For this review, take the finished solid that the model builds, in its own axes (mm). Face numbers are marked on the shaded views. Coordinates: 2 decimals unless noted, no trailing zeros. Order: outer loops, then holes, each group sorted by start corner. A loop starts at its lowest first (then second) coordinate and runs counter-clockwise, first axis right, second up.
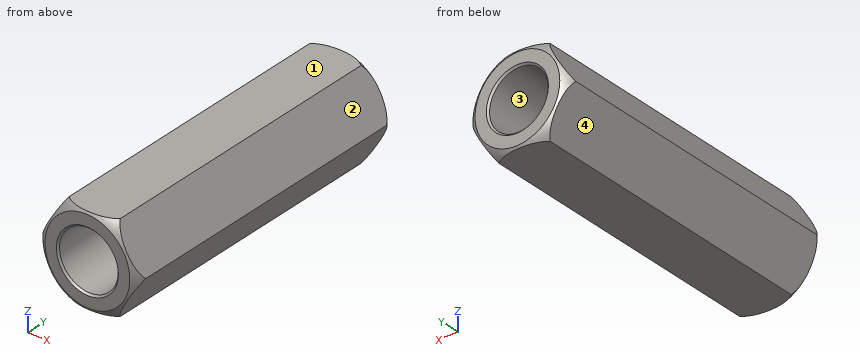
Autodesk Inventor part; units mm, degrees
ref_plane "YZ Plane" through (0, 0, 0) normal (1, 0, 0) x (0, 1, 0)
ref_plane "XZ Plane" through (0, 0, 0) normal (0, 1, 0) x (-1, 0, 0)
ref_plane "XY Plane" through (0, 0, 0) normal (0, 0, 1) x (1, 0, 0)
sketch "Sketch1" plane through (0, 0, 0) normal (0, 1, 0) x (-1, 0, 0)
  line L0 (-1.8331, -3.175) -> (-3.6662, 0)
  line L1 (-3.6662, 0) -> (-1.8331, 3.175)
  line L2 (-1.8331, 3.175) -> (1.8331, 3.175)
  line L3 (1.8331, 3.175) -> (3.6662, 0)
  line L4 (3.6662, 0) -> (1.8331, -3.175)
  line L5 (1.8331, -3.175) -> (-1.8331, -3.175)
  point P0 (0, 0)
  point P1 (0, 0)
  dimension "d0" = 6.35
extrude "Body" add sketch "Sketch1" along normal blind 22.225
sketch "Sketch2" plane through (0, 22.225, 0) normal (0, 1, 0) x (1, 0, 0)
  circle A0 centre (0, 0) radius 2.0955
  dimension "d3" = 4.191
extrude "Hole 2" cut sketch "Sketch2" against normal blind 12.7
sketch "Sketch3" plane through (0, 0, 0) normal (0, -1, 0) x (1, 0, 0)
  circle A0 centre (0, 0) radius 2.0955
  dimension "d6" = 4.191
extrude "Hole 1" cut sketch "Sketch3" against normal blind 12.7
chamfer "Hole 2 Chamfer 1" distance 0.127 distance2 0.1244 1 edges at (-2.0955, 22.225, 0) measured on face at (0.0842, 22.225, 2.8101)
chamfer "Hole 1 Chamfer 1" distance 0.127 distance2 0.1244 1 edges at (-2.0955, 0, 0) measured on face at (-0.0842, 0, 2.8101)
sketch "Sketch4" plane through (0, 0, 0) normal (0, 0, 1) x (1, 0, 0)
  line L0 (1.8331, 22.225) -> (-1.8331, 22.225)
  line L1 (0, 22.225) -> (-3.0353, 22.225)
  line L2 (-3.6662, 22.225) -> (-1.8331, 22.225)
  line L3 (-3.6662, 0) -> (-3.6662, 22.225)
  arc A0 (-3.0353, 22.225) -> (-3.6662, 21.59) centre (-2.2234, 20.7874) ccw
  line L4 (-3.6662, 21.59) -> (-6.3588, 24.1897)
  line L5 (-6.3588, 24.1897) -> (0, 22.225)
  line L6 (0, 22.225) -> (0, 75.889)
  point P0 (0, 0)
  dimension "d15" = 3.0353
  dimension "d16" = 1.651
  dimension "d17" = 0.635
revolve "Hole 2 Chamfer 2" cut sketch "Sketch4" angle 360 about axis through (0, 22.225, 0) along (0, 1, 0)
sketch "Sketch5" plane through (0, 0, 0) normal (0, 0, 1) x (1, 0, 0)
  line L0 (0, 0) -> (-3.0353, 0)
  line L1 (1.8331, 0) -> (-1.8331, 0)
  line L2 (-3.6662, 0) -> (-3.6662, 22.225)
  arc A0 (-3.6662, 0.635) -> (-3.0353, 0) centre (-2.2234, 1.4376) ccw
  line L3 (0, 0) -> (0, -2.1986)
  line L4 (-3.6662, 0.635) -> (-4.1154, -0.8715)
  line L5 (-4.1154, -0.8715) -> (0, 0)
  point P0 (-3.6662, 21.59)
  dimension "d19" = 3.0353
  dimension "d20" = 1.651
  dimension "d21" = 0.635
revolve "Hole 1 Chamfer 2" cut sketch "Sketch5" angle 360 about axis through (0, 0, 0) along (0, -1, 0)
chamfer "Hole 2 Chamfer 1 For Short" [suppressed]
sketch "Sketch7" plane through (0, 0, 0) normal (0, 0, 1) x (1, 0, 0)
  line L0 (0, 22.2254) -> (3.0353, 22.225)
  line L1 (3.6662, 22.225) -> (1.8331, 22.225)
  line L2 (3.6662, 0.635) -> (3.6662, 22.225)
  arc A0 (3.6662, 21.59) -> (3.0353, 22.225) centre (2.2234, 20.7874) ccw
  line L3 (3.6662, 21.59) -> (4.2663, 23.1282)
  line L4 (4.2663, 23.1282) -> (0, 22.2254)
  line L5 (0, 24.0311) -> (0, 22.2254)
  line L6 (1.8331, 22.225) -> (-1.8331, 22.225)
  point P0 (0, 0)
  point P1 (0, 22.225)
  dimension "d33" = 3.0353
  dimension "d34" = 1.651
  dimension "d35" = 0.635
revolve "Hole 2 Chamfer 2 For Short" [suppressed]
properties part number "Standoff .5" material "VEX Aluminum Alloy 5052-H32"
1. Take a section at B-B, the plane y = 5.5. Give the boundary of the cut face in (x, z) (1 decimal), plus the area to 3 significant figures.
Answer below:
outline: (-3.7, 0) - (-1.8, -3.2) - (1.8, -3.2) - (3.7, 0) - (1.8, 3.2) - (-1.8, 3.2) - close; hole circle Ø4.2 at (0, 0)
area: 21.1 mm2
2. Clearance check with flat-ended pins moving along their axes: pin 1 Ø4 at (x, y) = (-2.5, 15) entering from +Z (3 decimals); pin 2 Ø1.5 at (y, z) = (12, 1.5) entering from +X; pin 3 Ø3 at (y, z) = (8, -1) entering from +X. State where each tip first meets the part, or that it passes through.
Answer below:
pin 1: stops at z = 3.175
pin 2: stops at x = 3.23
pin 3: stops at x = 3.67
3. The part is to be moulded in two halves that separate along X. For the marked faces 1, 2, 3 and 4, say which applies: +X half, -X half, draft (parallel to the pull), parting line (faces both ways), or undercut.
Answer below:
face 1: draft
face 2: +X half
face 3: undercut
face 4: -X half
4. To check wall thickness, follow L1, parallel to Z at x = 0, y = 15.75 (1 decimal); L2, parallel to X at y = 19.25, z = -2.5; L3, parallel to Z at x = -1.5, y = 6 (3 decimals). State the ranges of each line that lie inside material, in increasing order.
Answer below:
L1: z = -3.2 to -2.1, 2.1 to 3.2
L2: x = -2.22 to 2.22
L3: z = -3.175 to -1.463, 1.463 to 3.175
